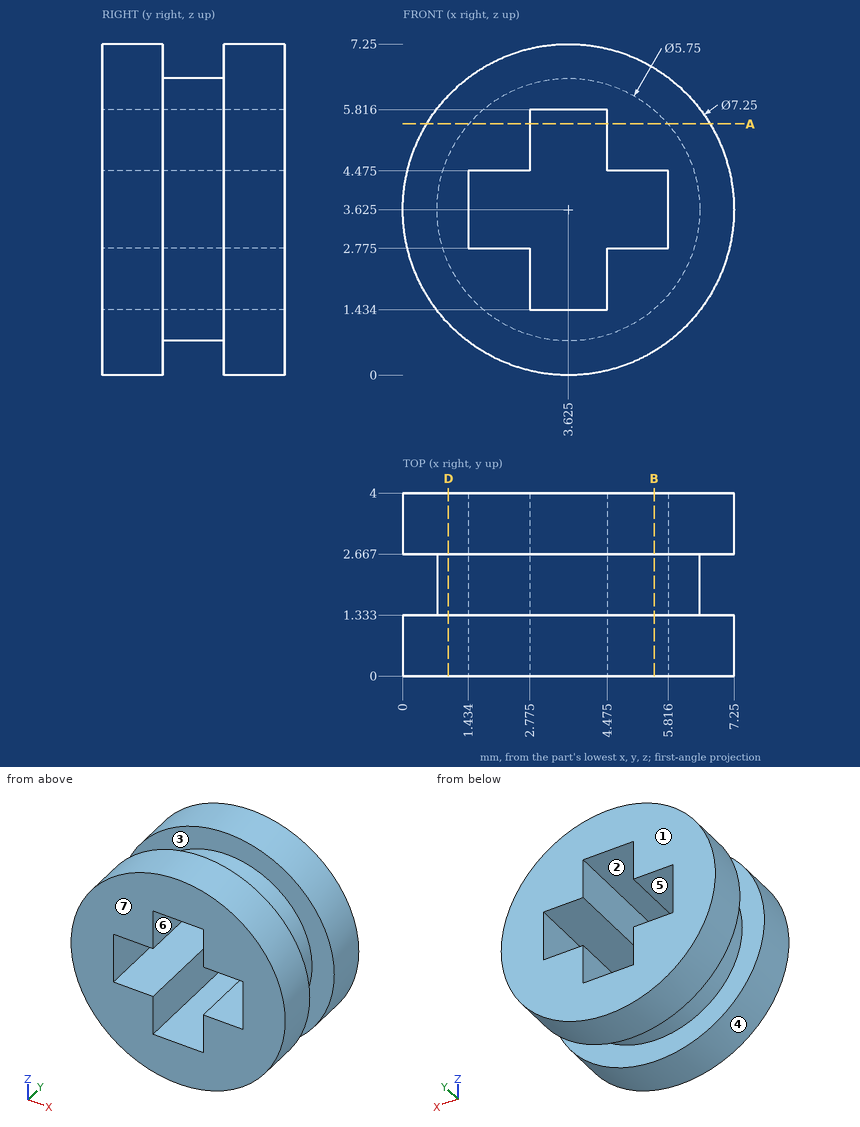
Verification items for this drawing (mm, ordinates from the low corner). A direction names the side the tool comes from. Give positions to 0.01 mm unless a question says otherwise; leave off trailing zeros. Order: outer loops, then holes, each group sorted by start corner. A loop starts at its lowest first (then second) coordinate and runs counter-clockwise, first axis right, second up.
1) Gauge pin test, flat ends, axial feed: pin 1 (4 mm diameter, centred on x = 1.5, z = 6, fed in from -Y); pin 2 (2 mm diameter, centred on y = 2.5, z = 6, fed in from +X); pin 3 (1 mm diameter, centred on x = 1.5, y = 3.5, fed in from -Z) (1 decimal); pin 4 (1.5 mm diameter, centred on x = 5.5, y = 3, fed in from -Z). Record the tip position at first contact, or that the pin passes through.
Results are:
pin 1: stops at y = 0
pin 2: stops at x = 6.97
pin 3: stops at z = 0.4
pin 4: stops at z = 0.18
2) Cross-section at B-B (x = 5.5). Record the boundary of the cut face in (y, z) (1 decimal).
Results are:
outline: (0, 0.5) - (1.3, 0.5) - (1.3, 1.4) - (2.7, 1.4) - (2.7, 0.5) - (4, 0.5) - (4, 2.8) - (0, 2.8) - close; (0, 4.5) - (4, 4.5) - (4, 6.7) - (2.7, 6.7) - (2.7, 5.8) - (1.3, 5.8) - (1.3, 6.7) - (0, 6.7) - close
3) Tool access check on the marked faces 1, 2 and 3. Record the directions out of +Z, -Z, +X, -X, +Y, -Y that give a thin tool (end or side, any length) a straight path to the whole face; none if there is none.
Results are:
face 1: +Z, -Z, +X, -X, +Y
face 2: +Y, -Y
face 3: none
4) Draft check along Z on the marked faces 4, 5, 6 and 7. Enter one of: released by +Z, released by -Z, zero draft, split by the parting line, or undercut.
Results are:
face 4: split by the parting line
face 5: undercut
face 6: undercut
face 7: zero draft
5) Cross-section at D-D (x = 1). Record the boundary of the cut face in (y, z) (1 decimal).
Results are:
outline: (0, 1.1) - (1.3, 1.1) - (1.3, 2.5) - (2.7, 2.5) - (2.7, 1.1) - (4, 1.1) - (4, 6.1) - (2.7, 6.1) - (2.7, 4.8) - (1.3, 4.8) - (1.3, 6.1) - (0, 6.1) - close
6) Material ranges on probe 1 along Z at (x, y) = (3.5, 0.65); probe 2 along Y at (x, z) = (2.5, 7); probe 3 along X at (y, z) = (2.15, 5.25) (1 decimal), recorded low to high.
Results are:
probe 1: z = 0 to 1.43, 5.82 to 7.25
probe 2: y = 0 to 1.33, 2.67 to 4
probe 3: x = 1.3 to 2.8, 4.5 to 6
7) Cross-section at A-A (z = 5.5). Record the boundary of the cut face in (x, y) (1 decimal).
Results are:
outline: (0.5, 0) - (2.8, 0) - (2.8, 4) - (0.5, 4) - (0.5, 2.7) - (1.4, 2.7) - (1.4, 1.3) - (0.5, 1.3) - close; (4.5, 0) - (6.7, 0) - (6.7, 1.3) - (5.8, 1.3) - (5.8, 2.7) - (6.7, 2.7) - (6.7, 4) - (4.5, 4) - close
